Part model, mm, in its own coordinate system. A direction names the side the tool comes from. Coordinates: 2 decimals unless noted, no trailing zeros. Loops run counter-clockwise (first coordinate to the right, second up) from the corner with the lowest first, then second, coordinate; pieces in that order, holes last. Notation, with made-up numbers: M 63,51 L 85,51 A35 cw 85,89 Z; hole C 89.25,52 d4. An arc over 180 degrees is marked long. Use a Markdown table: item, result. Add a question column.
1) Pin check, flat tips, straight feed: pin 1 Ø4 at (x, y) = (97.5, 4.5) entering from -Z; pin 2 Ø3 at (x, z) = (5.5, -62) entering from -Y; pin 3 Ø16.5 at (x, z) = (98, -49.5) entering from +Y; pin 4 Ø1.5 at (y, z) = (12, -2) entering from -X. Stop position of each tip, or through.
2) Pull direction X, two halves, no side cores. Call faces 1 (the cylindrical face through (85.89, 18.24, -86.05)), 2 (the cylindrical face through (97.23, 4.93, -54.57)), 3 (the flat face through (44, 18, -88.9)): released by +X, released by -X, zero draft, split by the parting line, or undercut.
3) Band-saw the part on A-A (x = 44.45). State how many separate pieces and enclosed holes the cut face has, plus the area to 3 significant figures.
4) Tool access for faces 4 (the flat face through (52.325, 14, 16)), 5 (the cylindrical face through (83.267, 9.86, -49.547)), 6 (the flat face through (-8, 5, -59.45)), 7 (the flat face through (22.325, 14, 16)): list every direction of +Z, -Z, +X, -X, +Y, -Y with a clear straight run to the whole face (end or side of a thin tool).
5) Band-saw the part on D-D (x = 96.4). List the corners of the cut face in (y, z), plus the area to 3 significant figures.
6) Band-saw the part on B-B (y = 14.5). List the corners of the cut face in (x, z), plus the area to 3 significant figures.
7) Wall check: probe 1 along Z at (x, y) = (39, 28.5); probe 2 along Z at (x, y) = (44, 8); probe 3 along X at (y, z) = (30.25, -44.45). Give the ranges that are in metal, low to high. Write a range as from..to.
8) Band-saw the part on C-C (z = -44.45). List the corners of the cut face in (x, y), plus the area to 3 significant figures.
from build123d import *

# Parameters (mm, degrees)
SKETCH1_W           = 88.9
SKETCH1_H           = 88.9
SKETCH1_R           = 39.15
BOSS_EXTRUDE1_DEPTH = 20
SKETCH2_W           = 88.9
SKETCH2_H           = 88.9
SKETCH2_R           = 33
BOSS_EXTRUDE3_DEPTH = 5
SKETCH3_W           = 88.9
SKETCH3_H           = 88.9
SKETCH3_R           = 39.15
BOSS_EXTRUDE4_DEPTH = 12
SKETCH4_W           = 15
SKETCH4_H           = 15
SKETCH4_R           = 2.75
BOSS_EXTRUDE5_DEPTH = 10
FILLET1_R           = 5
FILLET2_R           = 10
SKETCH5_W           = 30
SKETCH5_H           = 4
BOSS_EXTRUDE6_DEPTH = 15
SKETCH6_W           = 30
SKETCH6_H           = 31
SKETCH6_H_2         = 4
BOSS_EXTRUDE7_DEPTH = 5
FILLET3_R           = 3


with BuildPart() as part:
    # Sketch1 → Boss-Extrude1 (new body)
    with BuildSketch(Plane(origin=(0, 0, 0), x_dir=(1, 0, 0), z_dir=(0, 1, 0))):
        with Locations((44.45, 44.45)):
            Rectangle(SKETCH1_W, SKETCH1_H)
        with Locations(Location((44.45, 44.45, 0), (0, 0, 270))):
            Circle(SKETCH1_R, mode=Mode.SUBTRACT)
    extrude(amount=BOSS_EXTRUDE1_DEPTH)

    # Sketch2 → Boss-Extrude3 (add)
    with BuildSketch(Plane(origin=(0, 20, 0), x_dir=(1, 0, 0), z_dir=(0, 1, 0))):
        with Locations((44.45, 44.45)):
            Rectangle(SKETCH2_W, SKETCH2_H)
        with Locations(Location((44.45, 44.45, 0), (0, 0, 270))):
            Circle(SKETCH2_R, mode=Mode.SUBTRACT)
    extrude(amount=BOSS_EXTRUDE3_DEPTH)

    # Sketch3 → Boss-Extrude4 (add)
    with BuildSketch(Plane(origin=(0, 25, 0), x_dir=(1, 0, 0), z_dir=(0, 1, 0))):
        with Locations((44.45, 44.45)):
            Rectangle(SKETCH3_W, SKETCH3_H)
        with Locations(Location((44.45, 44.45, 0), (0, 0, 270))):
            Circle(SKETCH3_R, mode=Mode.SUBTRACT)
    extrude(amount=BOSS_EXTRUDE4_DEPTH)

    # Sketch4 → Boss-Extrude5 (add)
    # profile 1 of 4: a face of its own
    with BuildSketch(Plane.XZ):
        with Locations((-7.5, -36.95)):
            Rectangle(SKETCH4_W, SKETCH4_H)
        with Locations(Location((-7.5, -36.95, 0), (0, 0, 270))):
            Circle(SKETCH4_R, mode=Mode.SUBTRACT)
    # profile 2 of 4: a face of its own
    with BuildSketch(Plane.XZ):
        with Locations((-7.5, -51.95)):
            Rectangle(SKETCH4_W, SKETCH4_H)
        with Locations(Location((-7.5, -51.95, 0), (0, 0, 270))):
            Circle(SKETCH4_R, mode=Mode.SUBTRACT)
    # profile 3 of 4: a face of its own
    with BuildSketch(Plane.XZ):
        with Locations((96.4, -36.95)):
            Rectangle(SKETCH4_W, SKETCH4_H)
        with Locations(Location((96.4, -36.95, 0), (0, 0, 270))):
            Circle(SKETCH4_R, mode=Mode.SUBTRACT)
    # profile 4 of 4: a face of its own
    with BuildSketch(Plane.XZ):
        with Locations((96.4, -51.95)):
            Rectangle(SKETCH4_W, SKETCH4_H)
        with Locations(Location((96.4, -51.95, 0), (0, 0, 270))):
            Circle(SKETCH4_R, mode=Mode.SUBTRACT)
    extrude(amount=-BOSS_EXTRUDE5_DEPTH)

    # Fillet1
    fillet1_edges = [part.edges().sort_by_distance(p)[0] for p in [
        (-15, 5, -59.45),
        (-15, 5, -29.45),
        (0, 5, -29.45),
        (0, 5, -59.45),
        (88.9, 5, -59.45),
        (88.9, 5, -29.45),
        (103.9, 5, -29.45),
        (103.9, 5, -59.45),
    ]]
    fillet(fillet1_edges, radius=FILLET1_R)

    # Fillet2
    fillet2_edges = [part.edges().sort_by_distance(p)[0] for p in [
        (0, 18.5, 0),
        (0, 18.5, -88.9),
        (88.9, 18.5, -88.9),
        (88.9, 18.5, 0),
    ]]
    fillet(fillet2_edges, radius=FILLET2_R)

    # Sketch5 → Boss-Extrude6 (add)
    with BuildSketch(Plane.XY):
        with Locations((37.32503103, 2)):
            Rectangle(SKETCH5_W, SKETCH5_H)
    extrude(amount=BOSS_EXTRUDE6_DEPTH)

    # Sketch6 → Boss-Extrude7 (add)
    # profile 1 of 2: a face of its own
    with BuildSketch(Plane.XY.offset(15)):
        with Locations((37.32503103, 19.5)):
            Rectangle(SKETCH6_W, SKETCH6_H)
        with BuildLine():
            ThreePointArc((25.32503103, 8.25), (23.57503103, 10), (25.32503103, 11.75))
            Line((25.32503103, 11.75), (49.32503103, 11.75))
            ThreePointArc((49.32503103, 11.75), (50.562467897, 11.237436867), (51.07503103, 10))
            ThreePointArc((51.07503103, 10), (50.562467897, 8.762563133), (49.32503103, 8.25))
            Line((49.32503103, 8.25), (25.32503103, 8.25))
        make_face(mode=Mode.SUBTRACT)
        with BuildLine():
            ThreePointArc((25.32503103, 30.25), (23.57503103, 32), (25.32503103, 33.75))
            Line((25.32503103, 33.75), (49.32503103, 33.75))
            ThreePointArc((49.32503103, 33.75), (50.562467897, 33.237436867), (51.07503103, 32))
            ThreePointArc((51.07503103, 32), (50.562467897, 30.762563133), (49.32503103, 30.25))
            Line((49.32503103, 30.25), (25.32503103, 30.25))
        make_face(mode=Mode.SUBTRACT)
    # profile 2 of 2: a face of its own
    with BuildSketch(Plane.XY.offset(15)):
        with Locations((37.32503103, 2)):
            Rectangle(SKETCH6_W, SKETCH6_H_2)
    extrude(amount=BOSS_EXTRUDE7_DEPTH)

    # Fillet3
    fillet3_edges = [part.edges().sort_by_distance(p)[0] for p in [
        (22.32503103, 35, 17.5),
        (52.32503103, 35, 17.5),
        (37.32503103, 0, 20),
    ]]
    fillet(fillet3_edges, radius=FILLET3_R)


solid = part.part
Entries:
| question | item | result |
|---|---|---|
| 1 | pin 1 | z = -59.45 |
| 1 | pin 2 | y = 0 |
| 1 | pin 3 | y = 10 |
| 1 | pin 4 | x = 3.11 |
| 2 | face 1 | released by +X |
| 2 | face 2 | undercut |
| 2 | face 3 | zero draft |
| 3 | separate pieces | 4 |
| 3 | enclosed holes | 0 |
| 3 | area | 652 mm2 |
| 4 | face 4 | +Z, +X, +Y, -Y |
| 4 | face 5 | -Y |
| 4 | face 6 | -Z, -X, +Y, -Y |
| 4 | face 7 | +Z, -X, +Y, -Y |
| 5 | outline | M 0,-59.45 L 10,-59.45 L 10,-54.7 L 0,-54.7 Z; M 0,-49.2 L 10,-49.2 L 10,-39.7 L 0,-39.7 Z; M 0,-34.2 L 10,-34.2 L 10,-29.45 L 0,-29.45 Z |
| 5 | area | 190 mm2 |
| 6 | outline | M 0,-78.9 A10 ccw 10,-88.9 L 78.9,-88.9 A10 ccw 88.9,-78.9 L 88.9,-10 A10 ccw 78.9,0 L 10,0 A10 ccw 0,-10 Z; M 22.33,15 L 52.33,15 L 52.33,20 L 22.33,20 Z; hole C 44.45,-44.45 d78.3 |
| 6 | area | 3,150 mm2 |
| 7 | probe 1 | -88.9..-83.22, -5.68..0, 15..20 |
| 7 | probe 2 | -88.9..-83.6, -5.3..0, 15..20 |
| 7 | probe 3 | 0..5.3, 83.6..88.9 |
| 8 | outline | M -15,0 L 5.3,0 L 5.3,20 L 11.45,20 L 11.45,25 L 5.3,25 L 5.3,37 L 0,37 L 0,10 L -15,10 Z; M 77.45,20 L 83.6,20 L 83.6,0 L 103.9,0 L 103.9,10 L 88.9,10 L 88.9,37 L 83.6,37 L 83.6,25 L 77.45,25 Z |
| 8 | area | 754 mm2 |
